CAD build for the part. Positions are in the model's coordinates, mm. A direction names the side the tool comes from. Round coordinates to 2 decimals unless told otherwise and drop trailing zeros. Loops run counter-clockwise (first coordinate to the right, second up) from the corner with the lowest first, then second, coordinate; pieces in that order, holes last.
```python
from build123d import *

# Parameters (mm, degrees)
F0_R     = 10.541
F1_DEPTH = 25.4
F2_R     = 8.001
F3_DEPTH = 22.86
F4_W     = 2.54
F4_H     = 2.54
F5_DEPTH = 22.86


with BuildPart() as f1:
    # F0 (on Top) → F1 (new body)
    with BuildSketch(Plane.XY):
        Circle(F0_R)
    extrude(amount=F1_DEPTH)

    # F2 (on face) → F3 (cut)
    with BuildSketch(Plane.XY.offset(25.4)):
        Circle(F2_R)
    extrude(amount=-F3_DEPTH, mode=Mode.SUBTRACT)

    # F4 (on face) → F5 (join)
    with BuildSketch(Plane.XY.offset(2.54)):
        Rectangle(F4_W, F4_H)
        with BuildLine():
            Line((1.27, 1.27), (1.27, -1.27))
            Line((1.27, -1.27), (7.8995633424, -1.27))
            ThreePointArc((7.8995633424, -1.27), (7.9756005198, -0.6370222515), (8.001, 0))
            ThreePointArc((8.001, 0), (7.9756005198, 0.6370222515), (7.8995633424, 1.27))
            Line((7.8995633424, 1.27), (1.27, 1.27))
        make_face()
        with BuildLine():
            Line((-1.27, -1.27), (-1.27, -7.8995633424))
            ThreePointArc((-1.27, -7.8995633424), (0, -8.001), (1.27, -7.8995633424))
            Line((1.27, -7.8995633424), (1.27, -1.27))
            Line((1.27, -1.27), (-1.27, -1.27))
        make_face()
        with BuildLine():
            Line((-7.8995633424, -1.27), (-1.27, -1.27))
            Line((-1.27, -1.27), (-1.27, 1.27))
            Line((-1.27, 1.27), (-7.8995633424, 1.27))
            ThreePointArc((-7.8995633424, 1.27), (-8.001, 0), (-7.8995633424, -1.27))
        make_face()
        with BuildLine():
            Line((-1.27, 7.8995633424), (-1.27, 1.27))
            Line((-1.27, 1.27), (1.27, 1.27))
            Line((1.27, 1.27), (1.27, 7.8995633424))
            ThreePointArc((1.27, 7.8995633424), (0, 8.001), (-1.27, 7.8995633424))
        make_face()
    extrude(amount=F5_DEPTH)


solid = f1.part
```
Item 1: Two-plate mould, pull along Y, no slides. Class faces 3 (the flat face through (4, 4, 2.54)), 4 (the cylindrical face through (10.054, 3.166, 12.522)), 5 (the flat face through (0, 0, 25.4)), 6 (the flat face through (-5, -1.27, 14)): released by +Y, released by -Y, zero draft, split by the parting line, or undercut.
Answers follow:
face 3: undercut
face 4: split by the parting line
face 5: zero draft
face 6: undercut
Item 2: Probe line 1 (Y direction, x = 3.25, z = 6.5); line 2 (X direction, y = 4, z = 20.5); line 3 (X direction, y = 2.5, z = 23). List the from-to ranges inside material, lowest first.
Answers follow:
line 1: y = -10.03 to -7.31, -1.27 to 1.27, 7.31 to 10.03
line 2: x = -9.75 to -6.93, -1.27 to 1.27, 6.93 to 9.75
line 3: x = -10.24 to -7.6, -1.27 to 1.27, 7.6 to 10.24
Item 3: Flat gauge pins, fed straight in: P1, Ø2, axis at x = -5, y = -6, coming from the +Z side; P2, Ø7.5, axis at x = 5.5, z = 16.5, coming from the -Y side; P3, Ø4, axis at y = 4, z = 8, coming from the -X side; P4, Ø5.5, axis at y = 6, z = 19, coming from the +X side. Where does each tip first touch, or does it go through?
Answers follow:
P1: stops at z = 25.4
P2: stops at y = -10.39
P3: stops at x = -10.35
P4: stops at x = 10.03
Item 4: 3-axis set-ups, long thin cutter, end or side, ignore diameter. For faces 1 (the flat face through (-5, 1.27, 14)), 2 (the flat face through (0, 0, 0)): which of +Z, -Z, +X, -X, +Y, -Y reach the whole face in a straight line?
Answers follow:
face 1: +Z
face 2: -Z, +X, -X, +Y, -Y
Item 5: Cut at C-C, the plane y = 2. Give the cut face in (x, z).
Answers follow:
outline: (-10.35, 0) - (10.35, 0) - (10.35, 25.4) - (7.75, 25.4) - (7.75, 2.54) - (1.27, 2.54) - (1.27, 25.4) - (-1.27, 25.4) - (-1.27, 2.54) - (-7.75, 2.54) - (-7.75, 25.4) - (-10.35, 25.4) - close
Item 6: Cut at B-B, the plane y = 6.5. Give the cut face in (x, z), plus the area to 3 significant figures.
Answers follow:
outline: (-8.3, 0) - (8.3, 0) - (8.3, 25.4) - (4.67, 25.4) - (4.67, 2.54) - (1.27, 2.54) - (1.27, 25.4) - (-1.27, 25.4) - (-1.27, 2.54) - (-4.67, 2.54) - (-4.67, 25.4) - (-8.3, 25.4) - close
area: 266 mm2
Item 7: Cut at A-A, the plane z = 4. Give the cut face in (x, y).
Answers follow:
outline: circle Ø21.08 at (0, 0); hole (-7.9, -1.27) arc R8 ccw to (-1.27, -7.9) - (-1.27, -1.27) - close; hole (-7.9, 1.27) - (-1.27, 1.27) - (-1.27, 7.9) arc R8 ccw to start; hole (1.27, -7.9) arc R8 ccw to (7.9, -1.27) - (1.27, -1.27) - close; hole (1.27, 1.27) - (7.9, 1.27) arc R8 ccw to (1.27, 7.9) - close
